Source: CAD feature listing. Evaluate the final solid. Frame: model axes, mm. A direction names the side the tool comes from. Coordinates: 2 decimals unless noted, no trailing zeros. Order: outer loops, then holes, each group sorted by start corner. A loop starts at its lowest first (then second) coordinate and runs counter-clockwise, first axis right, second up. Notation, with made-up numbers: (81.25, 15.25) -> (135.25, 15.25) arc R23 cw to (135.25, 31.25) -> close; hole circle Ø9 at (50, 50.5). An arc over 180 degrees is marked (long way). Write item = value, one per line. Start each with the question number.
Item 1: Set-up query: faces 3 (the cylindrical face through (32.87, 2.44, -0.54)), 4 (the flat face through (5.311, 4, 5)). Return all of +Z, -Z, +X, -X, +Y, -Y with unobstructed straight access to the full face (end or side cutting, diameter ignored); none if empty.
Item 2: Mould query, pull axis Z, two halves, no side actions, for faces 1 (the flat face through (-9.689, 2, 2)), 2 (the flat face through (5.311, 4, -5)). Classes: released by +Z, released by -Z, zero draft, split by the parting line, or undercut.
Item 3: Contact query for flat-ended pins moving along their axis: pin 1 (6 mm diameter, centred on y = 0, z = 0, fed in from +X); pin 2 (10 mm diameter, centred on y = -5, z = 5, fed in from +X); pin 3 (1.5 mm diameter, centred on y = 5.5, z = 6, fed in from +X); pin 4 (10 mm diameter, centred on y = 1, z = -1, fed in from +X). Output: stop coordinate, or through.
Item 4: Section query A-A (x = 8.5). Output: boundary loops of the cut face in (y, z), then the cut area to 3 significant figures.
Item 5: Ray query, line 1 along Z through (x, y) = (-0.5, 4); line 2 along Z through (x, y) = (-6, 4); line 3 along Y through (x, z) = (7.5, 0). Return the intervals inside material, ascending. Write a range as [from, to].
```python
from build123d import *

# Parameters (mm, degrees)
F2_R     = 1.5
F3_DEPTH = 15


with BuildPart() as f1:
    # F0 (on Front) → F1 (revolve)
    with BuildSketch(Plane.XZ):
        with BuildLine():
            add(Edge.make_bspline(
                [(10.6524407623, 9.5214215845), (16.9594295824, 6.846512057), (23.6366284889, 6.813516644), (48.4088717457, 6.4159839242), (61.3018820008, 8.0772608919)],
                knots=[0, 0, 0, 0, 0.3859038631, 1, 1, 1, 1], degree=3))
            ThreePointArc((10.6524407623, 9.5214215845), (0.6865334357, 14.2709717618), (-9.6892705187, 10.5))
            Line((-9.6892705187, 10.5), (-9.6892705187, 2.5))
            Line((-9.6892705187, 2.5), (12.2474487139, 2.5))
            Line((12.2474487139, 2.5), (74.2474487139, 2.5))
            Line((74.2474487139, 2.5), (80.4566636234, 6.848955093))
            ThreePointArc((80.4566636234, 6.848955093), (71.1861926887, 12.2493617225), (61.3018820008, 8.0772608919))
        make_face()
    revolve(axis=Axis((35, 0, 0), (1, 0, 0)))

    # F2 (on face) → F3 (cut)
    with BuildSketch(Plane(origin=(-9.6892705187, 0, 0), x_dir=(0, -1, 0), z_dir=(-1, 0, 0))):
        with Locations((-4, 5)):
            Circle(F2_R)
        with Locations((4, 5)):
            Circle(F2_R)
        with Locations((4, -5)):
            Circle(F2_R)
        with Locations((-4, -5)):
            Circle(F2_R)
    extrude(amount=-F3_DEPTH, mode=Mode.SUBTRACT)


solid = f1.part
```
Computed:
q1.face_3 = +X, -X
q1.face_4 = -X
q2.face_1 = zero draft
q2.face_2 = undercut
q3.pin_1 = 74.96
q3.pin_2 = 80.46
q3.pin_3 = 80.08
q3.pin_4 = 79.84
q4.outline = circle Ø22.97 at (0, 0); hole circle Ø5 at (0, 0)
q4.area = 395 mm^2
q5.line_1 = [-13.71, -6.5], [-3.5, 3.5], [6.5, 13.71]
q5.line_2 = [-12.33, -6.5], [-3.5, 3.5], [6.5, 12.33]
q5.line_3 = [-12.16, -2.5], [2.5, 12.16]
